Autodesk Inventor part; units mm, degrees
ref_plane "YZ Plane" through (0, 0, 0) normal (1, 0, 0) x (0, 1, 0)
ref_plane "XZ Plane" through (0, 0, 0) normal (0, 1, 0) x (-1, 0, 0)
ref_plane "XY Plane" through (0, 0, 0) normal (0, 0, 1) x (1, 0, 0)
sketch "草图1" plane through (0, 0, 0) normal (0, 0, 1) x (1, 0, 0)
  line L0 (0, 0) -> (4, 0)
  line L1 (4, 0) -> (4, 2.5)
  line L2 (4, 2.5) -> (0, 2.5)
  line L3 (0, 2.5) -> (0, 0)
  line L4 (0, 2.5) -> (0, 5.5)
  arc A0 (3, 2.5) -> (0, 5.5) centre (0, 2.5) ccw
  dimension "d0" = 4
  dimension "d1" = 2.5
  dimension "d2" = 3
revolve "旋转1" add sketch "草图1" angle 360 about axis through (0, 2.5, 0) along (0, -1, 0)
sketch "草图2" plane through (0, 0, 0) normal (0, -1, 0) x (1, 0, 0)
  circle A0 centre (0, 0) radius 4
  line L0 (3.63, 1.6802) -> (3.63, -1.6802)
  circle A1 centre (0, 0) radius 4
  line L1 (0, 0) -> (0, -4) construction
  line L2 (-3.63, 1.6802) -> (-3.63, -1.6802)
  dimension "d4" = 3.63
extrude "拉伸1" cut sketch "草图2" against normal through all contours A0 L0 | L2 A0
sketch "草图3" plane through (0, 0, 0) normal (0, -1, 0) x (1, 0, 0)
  circle A0 centre (0, 0) radius 3
  dimension "d7" = 6
extrude "拉伸2" add sketch "草图3" along normal blind 0.2
sketch "草图4" plane through (0, 0, 0) normal (0, 0, 1) x (1, 0, 0)
  line L0 (3.63, 0) -> (3.63, 2.5)
  line L1 (3.63, 2.5) -> (3.63, 0)
  line L2 (3.63, 1.5) -> (5.1, 1.5)
  line L3 (5.1, 1.5) -> (5.1, 1.3)
  line L4 (5.1, 1.3) -> (3.63, 1.3)
  line L5 (3.63, 1.3) -> (3.63, 1.5)
  line L6 (-3.63, 2.5) -> (3.63, 2.5)
  line L7 (5.1, 1.5) -> (4.9, 1.5)
  line L8 (4.9, 1.5) -> (4.9, 0)
  line L9 (4.9, 0) -> (5.1, 0)
  line L10 (5.1, 0) -> (5.1, 1.5)
  line L11 (7.2, 0) -> (7.2, -0.2) construction
  line L12 (7.2, -0.2) -> (4.9, 0)
  line L13 (7.2, 0) -> (5.1, 0.1826)
  line L14 (7.2, 0) -> (7.2, -0.2)
  point P0 (0, 0)
  point P1 (4.9, 1.3)
  dimension "d10" = 1.47
  dimension "d11" = 1
  dimension "d12" = 0.2
  dimension "d13" = 0.2
  dimension "d14" = 1.5
  dimension "d15" = 0.2
  dimension "d16" = 2.1
extrude "拉伸3" add sketch "草图4" along normal mid plane 3.8
sketch "草图5" plane through (3.63, 1.5, 1.9) normal (0, 1, 0) x (1, 0, 0)
  line L0 (0, 3.8) -> (0, 3.5802)
  line L1 (0, 0.2198) -> (0, 3.5802)
  line L2 (0, 0.2198) -> (0, 0)
  line L3 (1.47, 0) -> (0, 0)
  line L4 (1.47, 0) -> (1.47, 3.8)
  line L5 (0, 3.8) -> (1.47, 3.8)
  line L6 (1.47, 3.8) -> (1.47, 0)
  line L7 (3.57, 0) -> (1.47, 0)
  line L8 (3.57, 3.8) -> (3.57, 0)
  line L9 (1.47, 3.8) -> (3.57, 3.8)
  line L10 (3.57, 3.8) -> (1.97, 3.8)
  line L11 (1.97, 3.8) -> (1.97, 2.3)
  line L12 (1.97, 2.3) -> (3.57, 2.3)
  line L13 (3.57, 2.3) -> (3.57, 3.8)
  line L14 (0, 3.5802) -> (1.97, 3.5802) construction
  line L15 (3.57, 3.8) -> (3.57, 0)
  line L16 (1.97, 3.05) -> (3.57, 3.05) construction
  line L17 (1.97, 3.8) -> (1.7502, 3.5802)
  line L18 (1.7502, 3.5802) -> (0, 3.5802)
  line L19 (0, 2.5198) -> (1.97, 2.5198) construction
  line L20 (1.97, 2.3) -> (1.7502, 2.5198)
  line L21 (1.7502, 2.5198) -> (1.47, 2.5198)
  line L22 (1.47, 0) -> (1.47, 3.8)
  line L23 (1.27, 3.8) -> (1.27, 0)
  line L24 (1.47, 2.5198) -> (1.27, 2.5198)
  line L25 (0, 0.2198) -> (0, 0)
  line L26 (0, 0.2198) -> (1.27, 0.2198)
  point P0 (-3.63, 1.9)
  dimension "d19" = 1.6
  dimension "d20" = 1.5
  dimension "d21" = 45
extrude "拉伸4" cut sketch "草图5" against normal through all contours L5 L23 L18 L0 | L5 L4 L18 L23 | L26 L23 L3 L2 | L9 L17 L18 L4 | L23 L24 L4 L3 | L21 L20 L12 L8 L7 L4
pattern_circular "环形阵列1" count 2 over 360 about axis through (0, -10, 0) along (0, 1, 0) of "拉伸3", "拉伸4"
properties part number "COB5730"
Source: CAD feature listing. Evaluate the final solid. Frame: model axes, mm. A direction names the side the tool comes from. Give positions to 0.01 mm unless a question says otherwise; leave off trailing zeros. Write each loop counter-clockwise with the first axis right and the second up, starting at its lowest first coordinate (ties: lowest second). Pieces come first, ordered by that corner, then holes. Notation, with made-up numbers: (67, -37.5) - (74, -37.5) arc R25 ccw to (74, -19.5) - close; hole circle Ø11 at (42.5, 57). An arc over 180 degrees is marked (long way). One line per item, written item: value. Start each with the question number.
Q1. Section query B-B, the plane y = 0.95. Return the cut outline in (x, z).
Q2. Set-up query: faces 1 (the face through (-2, 0, 3)), 2 (the face through (-3.63, 2, 0)), 3 (the face through (-4.9, 1, 1)). Return all of +Z, -Z, +X, -X, +Y, -Y with unobstructed straight access to the full face (end or side cutting, diameter ignored); none if empty.
Q3. Section query C-C, the plane z = 0. Return the cut outline in (x, y), then the cut area to 3 significant figures.
Q4. Section query A-A, the plane x = 0. Return the cut outline in (y, z).
Q5. Draft query along X for faces 4 (the face through (4.9, 1, -1)), 5 (the face through (-5.1, 1, 1)), 6 (the face through (-2, 2.5, 3)). Return one class per face: +X half, -X half, draft (parallel to the pull), parting line (faces both ways), or undercut.
Q6. Section query D-D, the plane y = 1.85. Return the cut outline in (x, z), then the cut area to 3 significant figures.
Q7. First-contact query: pin 1 Ø2 at (x, z) = (-3.5, -2) entering from +Y; pin 2 Ø1 at (x, z) = (4, 0.5) entering from -Y; pin 3 Ø1.5 at (x, y) = (-3.5, 0.5) entering from +Z. Flat tips, straight axial feed; report the tip coordinate or a pass-through.
Q8. Material intervals for probe 1 along Y at (x, z) = (-2, 2.75); probe 2 along X at (y, z) = (2.3, -0.25); probe 3 along Z at (x, y) = (1.5, 1.5), sorted ascending. Write a range as from..to.
Answer:
1. outline: (-5.1, 0.62) - (-4.9, 0.62) - (-4.9, 1.68) - (-5.1, 1.68) - close; (-3.63, -1.68) arc R4 ccw to (3.63, -1.68) - (3.63, 1.68) arc R4 ccw to (-3.63, 1.68) - close; (4.9, -1.68) - (5.1, -1.68) - (5.1, -0.62) - (4.9, -0.62) - close
2. face 1: -Y
2. face 2: +Z, -Z, -X, +Y
2. face 3: +Z, -Z, -Y
3. outline: (-4.9, 1.3) - (-3.63, 1.3) - (-3.63, 0) - (-3, 0) - (-3, -0.2) - (3, -0.2) - (3, 0) - (3.63, 0) - (3.63, 1.3) - (4.9, 1.3) - (4.9, 1.5) - (3.63, 1.5) - (3.63, 2.5) - (3, 2.5) arc R3 ccw to (-3, 2.5) - (-3.63, 2.5) - (-3.63, 1.5) - (-4.9, 1.5) - close
3. area: 34.0 mm2
4. outline: (-0.2, -3) - (0, -3) - (0, -4) - (2.5, -4) - (2.5, -3) arc R3 ccw to (2.5, 3) - (2.5, 4) - (0, 4) - (0, 3) - (-0.2, 3) - close
5. face 4: undercut
5. face 5: -X half
5. face 6: draft
6. outline: (-3.63, -1.68) arc R4 ccw to (3.63, -1.68) - (3.63, 1.68) arc R4 ccw to (-3.63, 1.68) - close
6. area: 48.6 mm2
7. pin 1: stops at y = 2.5
7. pin 2: stops at y = 0
7. pin 3: stops at z = 2.9
8. probe 1: y = 0..2.5
8. probe 2: x = -3.63..3.63
8. probe 3: z = -3.71..3.71
